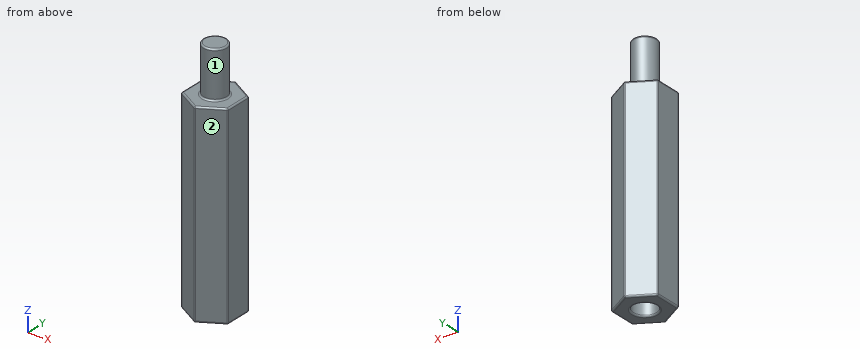
```python
from build123d import *

# Parameters (mm, degrees)
F1_DEPTH = 25
F2_R     = 1.5
F3_DEPTH = 6
F4_R     = 1.5
F5_DEPTH = 8
F6_R     = 0.2


with BuildPart() as f1:
    # F0 (on Top) → F1 (new body)
    with BuildSketch(Plane.XY):
        Polygon((3, 1.7320508076), (0, 3.4641016151), (-3, 1.7320508076), (-3, -1.7320508076), (0, -3.4641016151), (3, -1.7320508076), align=None)
    extrude(amount=F1_DEPTH)

    # F2 (on face) → F3 (join)
    with BuildSketch(Plane.XY.offset(25)):
        Circle(F2_R)
    extrude(amount=F3_DEPTH)

    # F4 (on face) → F5 (cut)
    with BuildSketch(Plane(origin=(0, 0, 0), x_dir=(1, 0, 0), z_dir=(0, 0, -1))):
        Circle(F4_R)
    extrude(amount=-F5_DEPTH, mode=Mode.SUBTRACT)

    # F6
    f6_edges = [f1.edges().sort_by_distance(p)[0] for p in [
        (1.5, -2.598076, 0),
        (-1.5, -2.598076, 0),
        (3, 0, 0),
        (-3, 0, 0),
        (1.5, 2.598076, 0),
        (-1.5, 2.598076, 0),
        (-1.5, 0, 0),
        (1.5, -2.598076, 25),
        (-1.5, -2.598076, 25),
        (3, 0, 25),
        (-3, 0, 25),
        (1.5, 2.598076, 25),
        (-1.5, 2.598076, 25),
        (-1.5, 0, 25),
        (-1.5, 0, 31),
        (-3, -1.732051, 12.5),
        (0, -3.464102, 12.5),
        (-3, 1.732051, 12.5),
        (0, 3.464102, 12.5),
        (3, 1.732051, 12.5),
        (3, -1.732051, 12.5),
    ]]
    fillet(f6_edges, radius=F6_R)


solid = f1.part
```
Here's how the part is built. I have some questions about the finished solid (model axes, mm). Face numbers are marked on the shaded views. A direction names the side the tool comes from. Give positions to 0.01 mm unless a question says otherwise; leave off trailing zeros. Write each loop counter-clockwise with the first axis right and the second up, starting at its lowest first coordinate (ties: lowest second). Pieces come first, ordered by that corner, then holes. Notation, with made-up numbers: M 29,18 L 72,18 A4 cw 72,25 Z; hole C 75,6 d8. An arc over 180 degrees is marked long. Put each result on its own line as item: value. Start each with the question number.
Item 1: On a 3-axis mill with a long thin cutter (end or side, diameter ignored), from which of +Z, -Z, +X, -X, +Y, -Y can I reach the whole of each face in a straight line? I mean the marked faces 1 and 2. Say none if no direction works.
Item 2: If we section it at A-A, the plane z = 7: Write out the boundary of the cut face in (x, y).
Item 3: I need wall thicknesses on L1, parallel to X at y = 0, z = 5.5; L2, parallel to Y at x = 0, z = 4; L3, parallel to Z at x = 2.25, y = 1.25. Which ranges of each line are inside material? Lowest first, please. Write a range as from..to.
Item 4: If we section it at B-B, the plane z = 16: Write out the boundary of the cut face in (x, y).
Item 5: If we section it at C-C, the plane y = 0: Write out the boundary of the cut face in (x, z), then the cut area to 3 significant figures.
Item 6: Will these pins go through, and if not, where does the flat tip stop? pin 1 (1.5 mm diameter, centred on x = 1.5, z = 5.5, fed in from +Y); pin 2 (3 mm diameter, centred on x = 2, z = 6, fed in from -Y).
Values:
1. face 1: +Z
1. face 2: +Z, -Z, +X, -Y
2. outline: M -3,-1.62 A0.2 ccw -2.9,-1.79 L -0.1,-3.41 A0.2 ccw 0.1,-3.41 L 2.9,-1.79 A0.2 ccw 3,-1.62 L 3,1.62 A0.2 ccw 2.9,1.79 L 0.1,3.41 A0.2 ccw -0.1,3.41 L -2.9,1.79 A0.2 ccw -3,1.62 Z; hole C 0,0 d3
3. L1: -3..-1.5, 1.5..3
3. L2: -3.43..-1.5, 1.5..3.43
3. L3: 0..25
4. outline: M -3,-1.62 A0.2 ccw -2.9,-1.79 L -0.1,-3.41 A0.2 ccw 0.1,-3.41 L 2.9,-1.79 A0.2 ccw 3,-1.62 L 3,1.62 A0.2 ccw 2.9,1.79 L 0.1,3.41 A0.2 ccw -0.1,3.41 L -2.9,1.79 A0.2 ccw -3,1.62 Z
5. outline: M -3,0.2 A0.2 ccw -2.8,0 L -1.7,0 A0.2 ccw -1.5,0.2 L -1.5,8 L 1.5,8 L 1.5,0.2 A0.2 ccw 1.7,0 L 2.8,0 A0.2 ccw 3,0.2 L 3,24.8 A0.2 ccw 2.8,25 L 1.7,25 A0.2 cw 1.5,25.2 L 1.5,30.8 A0.2 ccw 1.3,31 L -1.3,31 A0.2 ccw -1.5,30.8 L -1.5,25.2 A0.2 cw -1.7,25 L -2.8,25 A0.2 ccw -3,24.8 Z
5. area: 144 mm²
6. pin 1: y = 3.03
6. pin 2: y = -3.18
